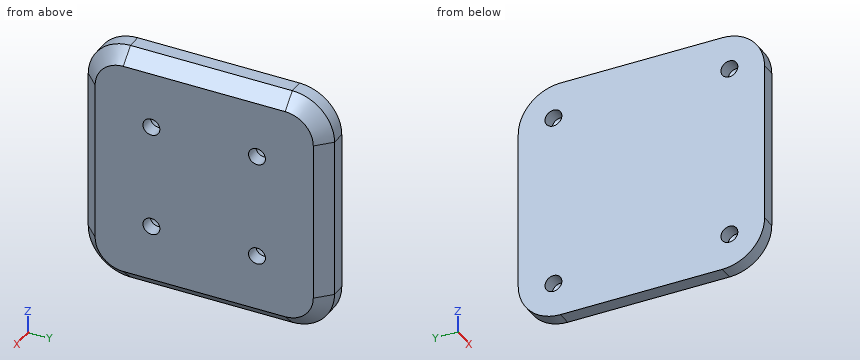
Autodesk Inventor part; units mm, degrees
ref_plane "YZ Plane" through (0, 0, 0) normal (1, 0, 0) x (0, 1, 0)
ref_plane "XZ Plane" through (0, 0, 0) normal (0, 1, 0) x (-1, 0, 0)
ref_plane "XY Plane" through (0, 0, 0) normal (0, 0, 1) x (1, 0, 0)
sketch "草圖1" plane through (0, 0, 0) normal (1, 0, 0) x (0, 1, 0)
  line L0 (-87.5, 87.5) -> (87.5, 87.5)
  line L1 (87.5, 87.5) -> (87.5, -87.5)
  line L2 (87.5, -87.5) -> (-87.5, -87.5)
  line L3 (-87.5, -87.5) -> (-87.5, 87.5)
  line L4 (-87.5, 87.5) -> (87.5, -87.5) construction
  line L5 (87.5, 87.5) -> (-87.5, -87.5) construction
  point P0 (0, 0)
  dimension "d0" = 175
  dimension "d1" = 175
extrude "擠出1" add sketch "草圖1" along normal blind 20
fillet "圓角1" radius 30 4 edges at (10, 87.5, 87.5) (10, -87.5, 87.5) (10, 87.5, -87.5) (10, -87.5, -87.5)
chamfer "倒角1" distance 10 angle 45 8 edges at (20, 0, 87.5) (20, -78.7132, 78.7132) (20, -87.5, 0) (20, -78.7132, -78.7132) (20, 0, -87.5) (20, 78.7132, -78.7132) (20, 87.5, 0) (20, 78.7132, 78.7132)
sketch "草圖2" plane through (20, 0, 0) normal (1, 0, 0) x (0, 0, -1)
  line L0 (-37.5, -37.5) -> (37.5, -37.5)
  line L1 (37.5, -37.5) -> (37.5, 37.5)
  line L2 (37.5, 37.5) -> (-37.5, 37.5)
  line L3 (-37.5, 37.5) -> (-37.5, -37.5)
  line L4 (-37.5, -37.5) -> (37.5, 37.5) construction
  line L5 (37.5, -37.5) -> (-37.5, 37.5) construction
  point P0 (0, 0)
  dimension "d8" = 75
  dimension "d9" = 75
hole "孔1" at (20, 37.5, 37.5) at (20, 37.5, -37.5) at (20, -37.5, 37.5) at (20, -37.5, -37.5) direction (-1, 0, 0) diameter 12 depth 10 tip angle 118
sketch "草圖3" plane through (0, 0, 0) normal (-1, 0, 0) x (0, 0, 1)
  arc A0 (-87.5, -57.5) -> (-57.5, -87.5) centre (-57.5, -57.5) ccw
  line L0 (-57.5, -87.5) -> (57.5, -87.5)
  arc A1 (57.5, -87.5) -> (87.5, -57.5) centre (57.5, -57.5) ccw
  line L1 (87.5, -57.5) -> (87.5, 57.5)
  arc A2 (87.5, 57.5) -> (57.5, 87.5) centre (57.5, 57.5) ccw
  line L2 (57.5, 87.5) -> (-57.5, 87.5)
  arc A3 (-57.5, 87.5) -> (-87.5, 57.5) centre (-57.5, 57.5) ccw
  line L3 (-87.5, 57.5) -> (-87.5, -57.5)
  line L4 (62.5, 62.5) -> (-62.5, 62.5)
  line L5 (-62.5, 62.5) -> (-62.5, -62.5)
  line L6 (-62.5, -62.5) -> (62.5, -62.5)
  line L7 (62.5, -62.5) -> (62.5, 62.5)
  line L8 (62.5, 62.5) -> (-62.5, -62.5) construction
  line L9 (-62.5, 62.5) -> (62.5, -62.5) construction
  point P0 (0, 0)
  dimension "d17" = 125
  dimension "d18" = 125
hole "孔2" at (0, -62.5, 62.5) at (0, -62.5, -62.5) at (0, 62.5, -62.5) at (0, 62.5, 62.5) direction (1, 0, 0) diameter 12 depth 10 tip angle 118
properties part number "exercise3-1-4"
The listing builds one solid part. Answer for the finished solid, in the listing's coordinates (mm). Coordinates: 2 decimals unless noted, no trailing zeros. Loops run counter-clockwise (first coordinate to the right, second up) from the corner with the lowest first, then second, coordinate; pieces in that order, holes last. Notation, with made-up numbers: M 70.5,19.25 L 128.5,19.25 A10 cw 128.5,34.25 Z; hole C 4,-0.5 d11. An arc over 180 degrees is marked long. Answer as a JSON object with one key per item and string values. Group by question number.
Item 1: Consider L1, parallel to Z at x = 2, y = 62.5; L2, parallel to Y at x = 14.5, z = -37.5. Determine where each line is inside the solid, lowest interval first.
Item 2: Section D-D (x = 17) is taken. Write down the section's boundary in (y, z), and give its area (3 significant figures).
Item 3: Each of these flat-tipped pins is pushed along its axis until it touches: P1, Ø11, axis at y = -37.5, z = -37.5, coming from the +X side; P2, Ø1, axis at y = -68.5, z = 15, coming from the -X side; P3, Ø1, axis at x = 16.5, y = -14.5, coming from the +Z side; P4, Ø2, axis at x = 17, y = 36, coming from the -Z side. Where does it stop, or does it pass through?
Item 4: Section A-A (x = 4.25) is taken. Write down the section's boundary in (y, z), and give its area (3 significant figures).
Item 5: Section B-B (z = 18) is taken. Write down the section's boundary in (x, y).
Solved:
{
 "1": {"L1": "z = -87.08 to -68.5, -56.5 to 56.5, 68.5 to 87.08", "L2": "y = -83 to -43.5, -31.5 to 31.5, 43.5 to 83"},
 "2": {"outline": "M -80.5,-57.5 A23 ccw -57.5,-80.5 L 57.5,-80.5 A23 ccw 80.5,-57.5 L 80.5,57.5 A23 ccw 57.5,80.5 L -57.5,80.5 A23 ccw -80.5,57.5 Z; hole C -37.5,-37.5 d12; hole C -37.5,37.5 d12; hole C 37.5,-37.5 d12; hole C 37.5,37.5 d12", "area": "25,000 mm2"},
 "3": {"P1": "stops at x = 9.7", "P2": "stops at x = 0", "P3": "stops at z = 81.5", "P4": "stops at z = -81.5"},
 "4": {"outline": "M -87.5,-57.5 A30 ccw -57.5,-87.5 L 57.5,-87.5 A30 ccw 87.5,-57.5 L 87.5,57.5 A30 ccw 57.5,87.5 L -57.5,87.5 A30 ccw -87.5,57.5 Z; hole C -62.5,-62.5 d12; hole C -62.5,62.5 d12; hole C 62.5,-62.5 d12; hole C 62.5,62.5 d12", "area": "29,400 mm2"},
 "5": {"outline": "M 0,-87.5 L 10,-87.5 L 20,-77.5 L 20,77.5 L 10,87.5 L 0,87.5 Z"}
}
